Read the model definition and answer for the solid it produces. Units are mm, in the model's axes. A direction names the side the tool comes from. Give positions to 0.01 mm unless a question says otherwise; leave off trailing zeros. Use a Markdown table: item, result. Add a question column.
1. A cutting plane is placed at A-A on x = 0. State how many separate pieces and enclosed holes the cut face has, and give its area (3 significant figures).
2. Flat-ended cylindrical pins translate along their axes: P1, Ø7.5, axis at x = 0.5, z = -24, coming from the -Y side; P2, Ø8, axis at x = 2, y = 18, coming from the +Z side; P3, Ø5, axis at x = -21, y = 19, coming from the -Z side; P4, Ø2, axis at y = 5.5, z = -11, coming from the -X side. Find the tip coordinate at first contact, or state that the pin passes through.
3. Which of the six approach directions +Z, -Z, +X, -X, +Y, -Y give full straight-line access (tool end or side, diameter ignored) to faces 1 (the cylindrical face through (-8, 15, -25)), 2 (the cylindrical face through (-25.847, 1.06, 0.147)), 3 (the cylindrical face through (0.221, 15.195, -20.814))?
4. For a pull along Z with two mould halves and no side action, classify faces 4 (the conical face through (11.34, 7.97, 20.65)), 5 (the conical face through (23.441, 6.877, -12.192)), 6 (the flat face through (6, 27.879, -13.3)) as released by +Z, released by -Z, zero draft, split by the parting line, or undercut.
5. Consider L1, parallel to Y at x = -17, z = -23; L2, parallel to Z at x = 23, y = 2.5; L3, parallel to X at y = 9.5, z = 11.5. Determine where each line is inside the solid, lowest interval first.
```python
from build123d import *

# Parameters (mm, degrees)
CBORE_FOR_M3_SBHCS1_D           = 3.4
CBORE_FOR_M3_SBHCS1_CBORE_D     = 6.7
CBORE_FOR_M3_SBHCS1_CBORE_DEPTH = 2.15
F_0_257_DIAMETER_HOLE1_D        = 6.5278
F_0_257_DIAMETER_HOLE1_DEPTH    = 6.35
F_0_257_DIAMETER_HOLE1_TIP      = 1.961148974


with BuildPart() as part:
    # Sketch1 → Revolve1 (revolve)
    with BuildSketch(Plane.XY, mode=Mode.PRIVATE) as revolve1_sk:
        Polygon((14.2875, 27.8791), (29, 27.8791), (29, 23.940468144), (26.25, 22.93955), (26.25, 6.93955), (29, 5.938631856), (29, 0), (14.2875, 0), align=None)
    revolve(revolve1_sk.sketch.rotate(Axis((0, 0, 0), (0, 1, 0)), 90), axis=Axis((0, 0, 0), (0, 1, 0)))

    # CBORE for M3 SBHCS1 (through all)
    with Locations(Plane.XZ):
        with Locations((0, 22.5), (0, -22.5), (22.5, 0), (-22.5, 0)):
            CounterBoreHole(CBORE_FOR_M3_SBHCS1_D / 2, CBORE_FOR_M3_SBHCS1_CBORE_D / 2, CBORE_FOR_M3_SBHCS1_CBORE_DEPTH)

    # F (0.257) Diameter Hole1
    with Locations(Plane.XZ):
        with Locations((-11.90625, 20.622229928), (-11.90625, -20.622229928), (11.90625, -20.622229928), (11.90625, 20.622229928)):
            Hole(F_0_257_DIAMETER_HOLE1_D / 2, depth=F_0_257_DIAMETER_HOLE1_DEPTH)
            with Locations((0, 0, -(F_0_257_DIAMETER_HOLE1_DEPTH + F_0_257_DIAMETER_HOLE1_TIP / 2))):  # 118° drill point
                Cone(0, F_0_257_DIAMETER_HOLE1_D / 2, F_0_257_DIAMETER_HOLE1_TIP, mode=Mode.SUBTRACT)


solid = part.part
```
Output values:
| question | item | result |
|---|---|---|
| 1 | separate pieces | 4 |
| 1 | enclosed holes | 0 |
| 1 | area | 523 mm² |
| 2 | P1 | y = 0 |
| 2 | P2 | z = 26.25 |
| 2 | P3 | z = -18.62 |
| 2 | P4 | x = -27.22 |
| 3 | face 1 | none |
| 3 | face 2 | -Y |
| 3 | face 3 | +Y, -Y |
| 4 | face 4 | undercut |
| 4 | face 5 | split by the parting line |
| 4 | face 6 | zero draft |
| 5 | L1 | 0 to 6.08, 23.8 to 27.88 |
| 5 | L2 | -17.66 to -1.62, 1.62 to 17.66 |
| 5 | L3 | -23.6 to -8.48, 8.48 to 23.6 |
